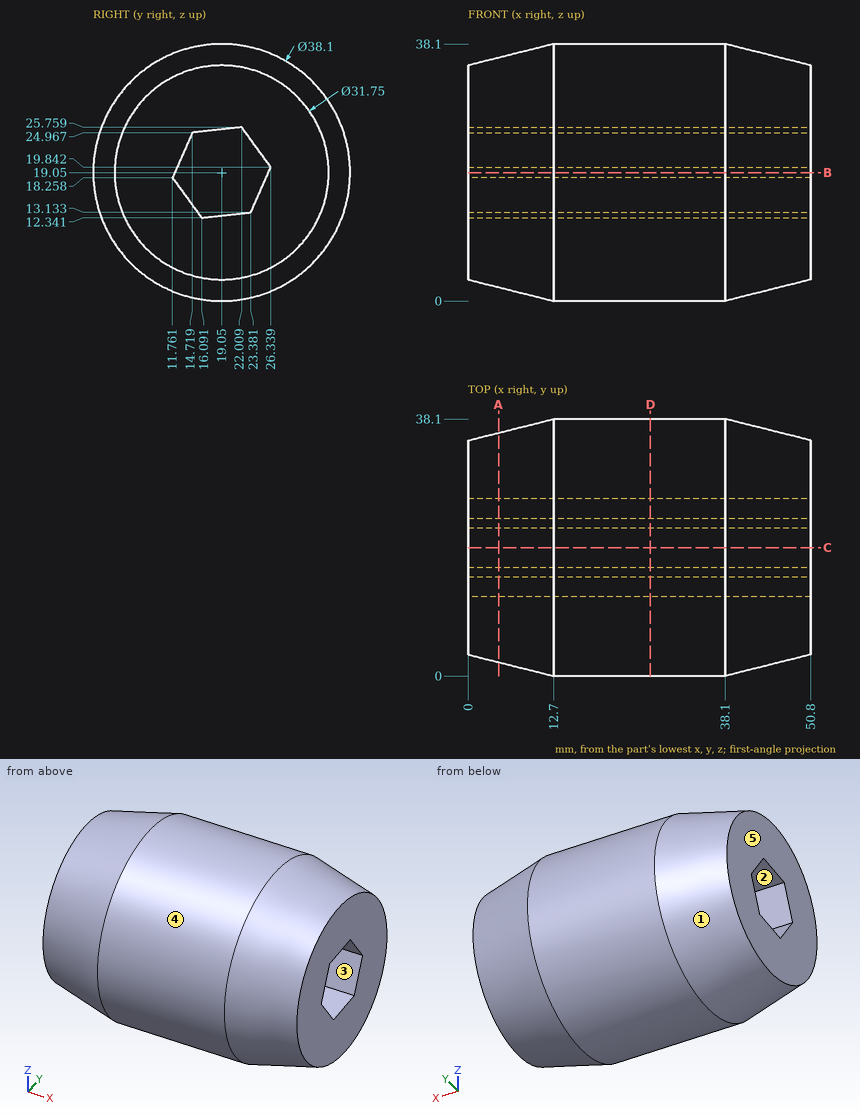
Here's the drawing with two shaded views (mm, measured from the low corner). I have some questions. A direction names the side the tool comes from. Coordinates: 2 decimals unless noted, no trailing zeros. Write each loop counter-clockwise with the first axis right and the second up, starting at its lowest first coordinate (ties: lowest second). Pieces come first, ordered by that corner, then holes. Notation, with made-up numbers: (-5.5, -40) -> (5.5, -40) arc R26 cw to (5.5, -23) -> close; hole circle Ø2 at (-8, 73.5). An arc over 180 degrees is marked (long way). Use a Markdown table: item, result. Add a question column.
(1) If we section it at B-B, the plane z = 19.05: Write out the boundary of the cut face in (x, y) (1 decimal).
(2) For the marked faces 1 and 2, which set-ups out of +Z, -Z, +X, -X, +Y, -Y let a thin tool reach every point of the face, with its end or its side?
(3) I'm going to push flat-ended pins straight in: P1, Ø3, axis at x = 32, y = 31, coming from the -Z side; P2, Ø12, axis at x = 36.5, z = 15.5, coming from the -Y side; P3, Ø5, axis at x = 36, y = 24.5, coming from the +Z side. Where does each tip first touch, or does it pass through?
(4) If we section it at A-A, the plane x = 4.5: Write out the boundary of the cut face in (y, z), and give its area (3 significant figures).
(5) If we section it at C-C, the plane y = 19.05: Write out the boundary of the cut face in (x, z) (1 decimal), and give its area (3 significant figures).
(6) We'd pull the mould along Z, two halves only. Please class the marked faces 3, 4 and 5: +Z half, -Z half, draft (parallel to the pull), parting line (faces both ways), or undercut.
(7) Please list where these lines run through material, in increasing order: line 1 (Z direction, x = 13, y = 18.5); line 2 (Y direction, x = 47.5, z = 19); line 3 (Z direction, x = 9, y = 18.5).
(8) If we section it at D-D, the plane x = 27: Write out the boundary of the cut face in (y, z).
Outcome:
| question | item | result |
|---|---|---|
| 1 | outline | (0, 3.2) -> (12.7, 0) -> (38.1, 0) -> (50.8, 3.2) -> (50.8, 12.1) -> (0, 12.1) -> close; (0, 26) -> (50.8, 26) -> (50.8, 34.9) -> (38.1, 38.1) -> (12.7, 38.1) -> (0, 34.9) -> close |
| 2 | face 1 | -X |
| 2 | face 2 | +X, -X |
| 3 | P1 | stops at z = 3.12 |
| 3 | P2 | stops at y = 0 |
| 3 | P3 | stops at z = 37.87 |
| 4 | outline | circle Ø34 at (19.05, 19.05); hole (11.76, 18.26) -> (16.09, 12.34) -> (23.38, 13.13) -> (26.34, 19.84) -> (22.01, 25.76) -> (14.72, 24.97) -> close |
| 4 | area | 768 mm^2 |
| 5 | outline | (0, 3.2) -> (12.7, 0) -> (38.1, 0) -> (50.8, 3.2) -> (50.8, 12.7) -> (0, 12.7) -> close; (0, 25.4) -> (50.8, 25.4) -> (50.8, 34.9) -> (38.1, 38.1) -> (12.7, 38.1) -> (0, 34.9) -> close |
| 5 | area | 1,210 mm^2 |
| 6 | face 3 | undercut |
| 6 | face 4 | parting line |
| 6 | face 5 | draft |
| 7 | line 1 | z = 0.01 to 12.6, 25.38 to 38.09 |
| 7 | line 2 | y = 2.35 to 12.09, 25.97 to 35.75 |
| 7 | line 3 | z = 0.93 to 12.6, 25.38 to 37.17 |
| 8 | outline | circle Ø38.1 at (19.05, 19.05); hole (11.76, 18.26) -> (16.09, 12.34) -> (23.38, 13.13) -> (26.34, 19.84) -> (22.01, 25.76) -> (14.72, 24.97) -> close |
